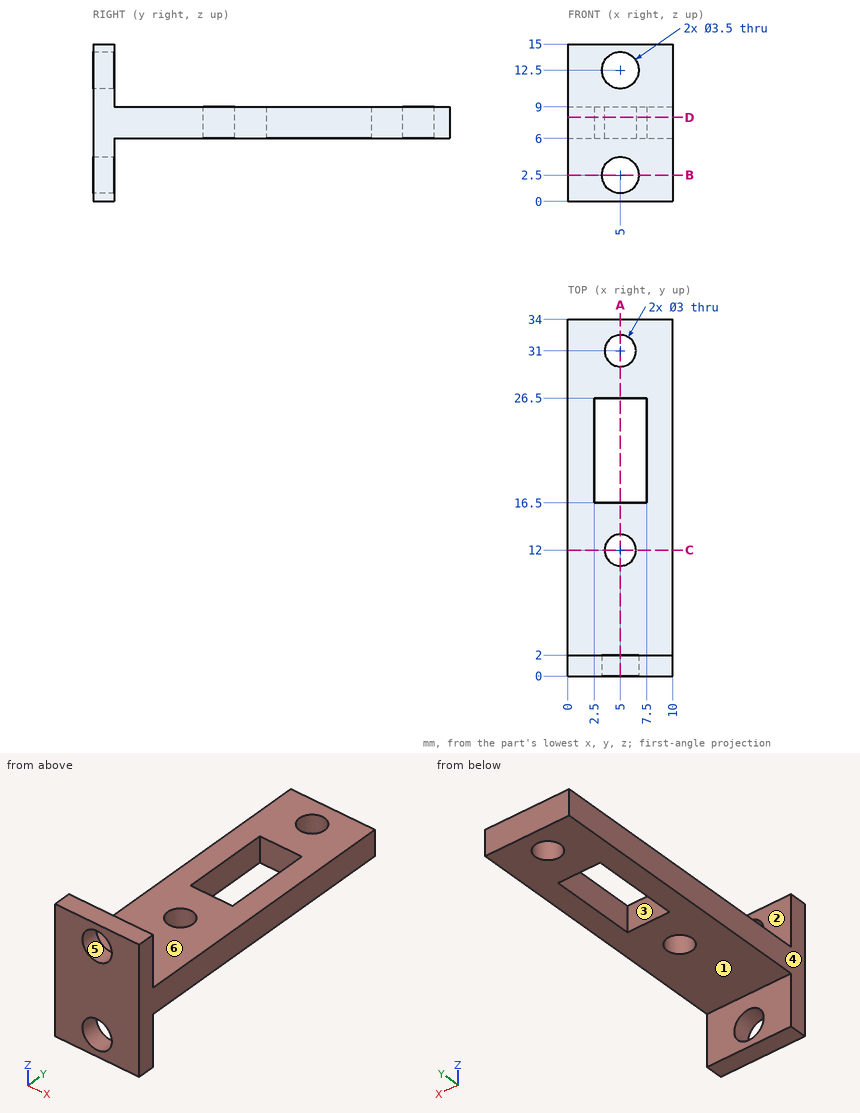
Drawing for the job (mm, zero at the part's lowest x, y, z). A direction names the side the tool comes from. Round coordinates to 2 decimals unless told otherwise and drop trailing zeros. Write each loop counter-clockwise with the first axis right and the second up, starting at its lowest first coordinate (ties: lowest second). Pieces come first, ordered by that corner, then holes. Notation, with made-up numbers: M -36.75,-6.75 L -5.75,-6.75 A24 ccw -5.75,24.25 Z; hole C 77.25,78 d9. An arc over 180 degrees is marked long. Put each result on its own line as item: value.
Item 1: Mould opens along X. For the marked faces 4, 5 and 6 say: +X half, -X half, draft (parallel to the pull), parting line (faces both ways), or undercut.
Responses:
face 4: -X half
face 5: undercut
face 6: draft
Item 2: Cut at D-D (z = 8). List the corners of the cut face in (x, y), and give its area (3 significant figures).
Responses:
outline: M 0,0 L 10,0 L 10,34 L 0,34 Z; hole M 2.5,16.5 L 7.5,16.5 L 7.5,26.5 L 2.5,26.5 Z; hole C 5,12 d3; hole C 5,31 d3
area: 276 mm²
Item 3: Tool access for the marked faces 1, 2 and 3: list every direction of +Z, -Z, +X, -X, +Y, -Y with a clear straight run to the whole face (end or side of a thin tool).
Responses:
face 1: -Z, +X, -X, +Y
face 2: +Z, +X, -X, +Y
face 3: +Z, -Z
Item 4: Cut at A-A (x = 5). List the corners of the cut face in (y, z).
Responses:
outline: M 0,0 L 2,0 L 2,0.75 L 0,0.75 Z; M 0,4.25 L 2,4.25 L 2,6 L 10.5,6 L 10.5,9 L 2,9 L 2,10.75 L 0,10.75 Z; M 0,14.25 L 2,14.25 L 2,15 L 0,15 Z; M 13.5,6 L 16.5,6 L 16.5,9 L 13.5,9 Z; M 26.5,6 L 29.5,6 L 29.5,9 L 26.5,9 Z; M 32.5,6 L 34,6 L 34,9 L 32.5,9 Z
Item 5: Probe L1, parallel to Y at x = 5, z = 7.9; L2, parallel to X at y = 0.8, z = 2.5; L3, parallel to Y at x = 3.25, z = 8.75. List the from-to ranges inside material, lowest first. Write a range as from..to.
Responses:
L1: 0..10.5, 13.5..16.5, 26.5..29.5, 32.5..34
L2: 0..3.25, 6.75..10
L3: 0..16.5, 26.5..34
Item 6: Flat gauge pins, fed straight in: P1, Ø5.5, axis at x = 5, z = 2.5, coming from the +Y side; P2, Ø5, axis at x = 2.5, y = 10, coming from the +Z side; P3, Ø3, axis at x = 6.5, y = 12, coming from the -Z side. Where does each tip first touch, or does it go through?
Responses:
P1: y = 2
P2: z = 9
P3: z = 6
Item 7: Cut at C-C (y = 12). List the corners of the cut face in (x, z), and give its area (3 significant figures).
Responses:
outline: M 0,6 L 3.5,6 L 3.5,9 L 0,9 Z; M 6.5,6 L 10,6 L 10,9 L 6.5,9 Z
area: 21.0 mm²
Item 8: Cut at B-B (z = 2.5). List the corners of the cut face in (x, y), and give its area (3 significant figures).
Responses:
outline: M 0,0 L 3.25,0 L 3.25,2 L 0,2 Z; M 6.75,0 L 10,0 L 10,2 L 6.75,2 Z
area: 13.0 mm²
